Design review of the part built by this model. Coordinates are the model's own, in mm. A direction names the side the tool comes from. Give positions to 0.01 mm unless a question says otherwise; leave off trailing zeros. Write each loop counter-clockwise with the first axis right and the second up, starting at its lowest first coordinate (ties: lowest second). Pieces come first, ordered by that corner, then holes. Notation, with made-up numbers: (79, 83) - (118, 83) arc R14 ccw to (118, 98) - close; hole circle Ø6 at (86.5, 39.5). An arc over 180 degrees is marked (long way). Write each question's results on one line, items separated by ' | '. Start each with the question number.
from build123d import *

# Parameters (mm, degrees)
SKETCH1_W               = 25.4
SKETCH1_H               = 35
BOSS_EXTRUDE1_DEPTH     = 12.7
FILLET1_R               = 0.05
SKETCH4_R               = 0.775
BOSS_EXTRUDE2_DEPTH     = 2
FILLET2_R               = 0.1
BOSS_EXTRUDE3_DEPTH     = 12.7
FILLET3_R               = 0.5
SKETCH12_W              = 28.953239704
SKETCH12_H              = 4.8
CUT_EXTRUDE6_DEPTH      = 13.7
CUT_EXTRUDE6_DEPTH_BACK = 3
SKETCH10_R              = 4.125
CUT_EXTRUDE1_DEPTH      = 3
CUT_EXTRUDE1_DEPTH_BACK = 13.7
SKETCH11_R              = 0.9
CUT_EXTRUDE3_DEPTH      = 3
CUT_EXTRUDE3_DEPTH_BACK = 5
FILLET4_R               = 0.5


with BuildPart() as part:
    # Sketch1 → Boss-Extrude1 (new body)
    with BuildSketch(Plane(origin=(0, 0, 0), x_dir=(1, 0, 0), z_dir=(0, 1, 0))):
        Rectangle(SKETCH1_W, SKETCH1_H)
    extrude(amount=BOSS_EXTRUDE1_DEPTH)

    # Sketch2 → Cut-Revolve1 (revolve, cut)
    with BuildSketch(Plane.XY):
        Polygon((3.75, 12.7), (3.75, 4.5), (2.05, 4.5), (2.05, 0), (0, 0), (0, 12.7), align=None)
    revolve(axis=Axis((0, 7.839551451, 0), (0, -1, 0)), mode=Mode.SUBTRACT)

    # Fillet1
    fillet1_edges = [part.edges().sort_by_distance(p)[0] for p in [
        (-3.75, 12.7, 0),
        (-3.75, 4.5, 0),
        (-2.05, 4.5, 0),
    ]]
    fillet(fillet1_edges, radius=FILLET1_R)

    # Sketch4 → Boss-Extrude2 (add)
    with BuildSketch(Plane.XZ):
        with Locations((0, 10.16)):
            Circle(SKETCH4_R)
        with Locations((0, -10.16)):
            Circle(SKETCH4_R)
    extrude(amount=BOSS_EXTRUDE2_DEPTH)

    # Fillet2
    fillet2_edges = [part.edges().sort_by_distance(p)[0] for p in [
        (-0.775, -2, 10.16),
        (-0.775, -2, -10.16),
    ]]
    fillet(fillet2_edges, radius=FILLET2_R)

    # Sketch9 → Boss-Extrude3 (add)
    with BuildSketch(Plane(origin=(0, 12.7, 0), x_dir=(1, 0, 0), z_dir=(0, 1, 0))):
        with BuildLine():
            Line((12.7, 17.5), (-12.7, 17.5))
            ThreePointArc((-12.7, 17.5), (0, 30.2), (12.7, 17.5))
        make_face()
    extrude(amount=-BOSS_EXTRUDE3_DEPTH)

    # Fillet3
    fillet3_edges = [part.edges().sort_by_distance(p)[0] for p in [
        (12.7, 12.7, 0),
        (-12.7, 12.7, 0),
        (0, 12.7, -30.2),
        (0, 0, -30.2),
        (12.7, 0, 0),
        (0, 0, 17.5),
        (-12.7, 0, 0),
    ]]
    fillet(fillet3_edges, radius=FILLET3_R)

    # Sketch12 → Cut-Extrude6 (cut, two sides)
    with BuildSketch(Plane(origin=(0, 0, 0), x_dir=(1, 0, 0), z_dir=(0, 1, 0))) as cut_extrude6_sk:
        with Locations((1.024131642, -15.1)):
            Rectangle(SKETCH12_W, SKETCH12_H)
    extrude(amount=CUT_EXTRUDE6_DEPTH, mode=Mode.SUBTRACT)
    extrude(cut_extrude6_sk.sketch, amount=-CUT_EXTRUDE6_DEPTH_BACK, mode=Mode.SUBTRACT)

    # Sketch10 → Cut-Extrude1 (cut, two sides)
    with BuildSketch(Plane.XZ) as cut_extrude1_sk:
        with Locations((0, -20)):
            Circle(SKETCH10_R)
    extrude(amount=CUT_EXTRUDE1_DEPTH, mode=Mode.SUBTRACT)
    extrude(cut_extrude1_sk.sketch, amount=-CUT_EXTRUDE1_DEPTH_BACK, mode=Mode.SUBTRACT)

    # Sketch11 → Cut-Extrude3 (cut, two sides)
    with BuildSketch(Plane.XZ) as cut_extrude3_sk:
        with Locations((0, -10.16)):
            Circle(SKETCH11_R)
        with Locations((0, 10.16)):
            Circle(SKETCH11_R)
    extrude(amount=CUT_EXTRUDE3_DEPTH, mode=Mode.SUBTRACT)
    extrude(cut_extrude3_sk.sketch, amount=-CUT_EXTRUDE3_DEPTH_BACK, mode=Mode.SUBTRACT)

    # Fillet4
    fillet4_edges = [part.edges().sort_by_distance(p)[0] for p in [
        (12.553553391, 0.146446609, 12.7),
        (-12.553553391, 12.553553391, 12.7),
        (-12.553553391, 0.146446609, 12.7),
        (12.553553391, 12.553553391, 12.7),
        (12.7, 6.35, 12.7),
        (0, 0, 12.7),
        (-12.7, 6.35, 12.7),
        (0, 12.7, 12.7),
    ]]
    fillet(fillet4_edges, radius=FILLET4_R)


solid = part.part
Q1. Insertion check: P1, Ø7, axis at x = 0, z = 0, coming from the +Y side; P2, Ø1.1, axis at x = 0, z = 10.16, coming from the -Y side. Each pin has a flat end and moves straight along its axis. Give the tip position at first contact, or say it passes through.
Q2. For line 1 along Z through (x, y) = (0, 3.05) (3 decimals); line 2 along Z through (x, y) = (0, 7) (3 decimals); line 3 along Z through (x, y) = (1.5, 1.5), list the stretches that pass through material, from the lowest coordinate up. Write a range as [from, to].
Q3. Machinability: for faces 1 (the face through (-3.746, 8.543, 0.165)), 2 (the face through (0, 5, 10)), 3 (the face through (0, 0, -9)), which of the approach directions +Z, -Z, +X, -X, +Y, -Y give a long, thin tool a straight path to every point of the face, cutting with its end or side? Answer none if there is none.
Q4. The part is to be moulded in two halves that separate along Z. For faces 4 (the face through (-0.195, 2.465, 9.281)), 5 (the face through (0, 12.7, -9)), 6 (the face through (2, 4.5, -2)), 7 (the face through (0, 6, 12.7)), say which applies: +Z half, -Z half, draft (parallel to the pull), parting line (faces both ways), or undercut.
Q5. Add section C-C on y = 10.75. State the section outline as (x, z) points (3 decimals), plus the area to 3 significant figures.
Q6. Add section B-B on z = 0. State the section outline as (x, y) points.
Q7. Add section A-A on x = 0. Count the separate pieces of the cut face and the enclosed holes in it, plus the area to 3 significant figures.
Q8. Add section D-D on z = 10.16. State the section outline as (x, y) points.
Result:
1) P1: stops at y = 4.5 | P2: stops at y = 5
2) line 1: z = [-30.2, -24.125], [-15.875, -11.06], [-9.26, -2.05], [2.05, 9.26], [11.06, 12.7] | line 2: z = [-30.2, -24.125], [-15.875, -3.75], [3.75, 12.7] | line 3: z = [-30.11, -23.84], [-16.16, -1.4], [1.4, 12.7]
3) face 1: +Y | face 2: -Y | face 3: +Z, -Z, +X, -X, -Y
4) face 4: undercut | face 5: draft | face 6: undercut | face 7: +Z half
5) outline: (-12.7, -17.5) arc R12.7 ccw to (12.7, -17.5) - (12.7, 12.2) arc R0.5 ccw to (12.2, 12.7) - (-12.2, 12.7) arc R0.5 ccw to (-12.7, 12.2) - close; hole circle Ø8.25 at (0, -20); hole circle Ø7.5 at (0, 0) | area: 923 mm²
6) outline: (-12.7, 0.5) arc R0.5 ccw to (-12.2, 0) - (-2.05, 0) - (-2.05, 4.45) arc R0.05 ccw to (-2.1, 4.5) - (-3.7, 4.5) arc R0.05 cw to (-3.75, 4.55) - (-3.75, 12.65) arc R0.05 ccw to (-3.8, 12.7) - (-12.2, 12.7) arc R0.5 ccw to (-12.7, 12.2) - close; (2.05, 0) - (12.2, 0) arc R0.5 ccw to (12.7, 0.5) - (12.7, 12.2) arc R0.5 ccw to (12.2, 12.7) - (3.8, 12.7) arc R0.05 ccw to (3.75, 12.65) - (3.75, 4.55) arc R0.05 cw to (3.7, 4.5) - (2.1, 4.5) arc R0.05 ccw to (2.05, 4.45) - close
7) separate pieces: 3 | enclosed holes: 0 | area: 342 mm²
8) outline: (-12.7, 0.5) arc R0.5 ccw to (-12.2, 0) - (-0.9, 0) - (-0.9, 5) - (0.9, 5) - (0.9, 0) - (12.2, 0) arc R0.5 ccw to (12.7, 0.5) - (12.7, 12.2) arc R0.5 ccw to (12.2, 12.7) - (-12.2, 12.7) arc R0.5 ccw to (-12.7, 12.2) - close
